from build123d import *

# Parameters (mm, degrees)
SKETCH1_R            = 21
BOSS_EXTRUDE1_DEPTH  = 3.5
SKETCH5_R            = 2.5
BOSS_EXTRUDE2_DEPTH  = 5
SKETCH6_R            = 5
SKETCH6_R_2          = 2.5
BOSS_EXTRUDE3_DEPTH  = 2.5
SKETCH7_R            = 17.5
BOSS_EXTRUDE4_DEPTH  = 0.75
SKETCH8_R            = 5
BOSS_EXTRUDE5_DEPTH  = 2.5
SKETCH10_R           = 1.125
SKETCH10_R_2         = 0.625
BOSS_EXTRUDE12_DEPTH = 0.5
CIRPATTERN1_COUNT    = 30


with BuildPart() as part:
    # Sketch1 → Boss-Extrude1 (new body)
    with BuildSketch(Plane(origin=(0, 0, 0), x_dir=(1, 0, 0), z_dir=(0, 1, 0))):
        with Locations(Location((0, 0, 0), (0, 0, 270))):
            Circle(SKETCH1_R)
    extrude(amount=BOSS_EXTRUDE1_DEPTH)

    # Sketch2 → Revolve3 (revolve)
    with BuildSketch(Plane.XY, mode=Mode.PRIVATE) as revolve3_sk:
        with BuildLine():
            Line((0, 3.5), (-20.5, 3.5))
            ThreePointArc((-20.5, 3.5), (-21.360863499, 9), (-20.5, 14.5))
            Line((-20.5, 14.5), (0, 14.5))
            Line((0, 14.5), (0, 3.5))
        make_face()
    revolve(revolve3_sk.sketch.rotate(Axis((0, 3.5, 0), (0, 1, 0)), 180), axis=Axis((0, 3.5, 0), (0, 1, 0)))

    # Sketch4 → Revolve4 (revolve)
    with BuildSketch(Plane.XY):
        with BuildLine():
            Line((0, 14.5), (21, 14.5))
            ThreePointArc((21, 14.5), (19.802282406, 20.151141203), (16, 24.5))
            Line((16, 24.5), (0, 24.5))
            Line((0, 24.5), (0, 14.5))
        make_face()
    revolve(axis=Axis((0, 14.5, 0), (0, 1, 0)))

    # Sketch5 → Boss-Extrude2 (add, symmetric)
    with BuildSketch(Plane.XY):
        with BuildLine():
            Line((0, 24.5), (10, 24.5))
            Line((10, 24.5), (10, 45.5))
            ThreePointArc((10, 45.5), (0, 55.5), (-10, 45.5))
            Line((-10, 45.5), (-10, 24.5))
            Line((-10, 24.5), (0, 24.5))
        make_face()
        with Locations((0, 45.5)):
            Circle(SKETCH5_R, mode=Mode.SUBTRACT)
    extrude(amount=BOSS_EXTRUDE2_DEPTH, both=True)

    # Sketch6 → Boss-Extrude3 (add, symmetric)
    with BuildSketch(Plane(origin=(0, 0, -5), x_dir=(-1, 0, 0), z_dir=(0, 0, -1))):
        with Locations(Location((0, 45.5, 0), (0, 0, 180))):
            Circle(SKETCH6_R)
        with Locations((0, 45.5)):
            Circle(SKETCH6_R_2, mode=Mode.SUBTRACT)
    extrude(amount=BOSS_EXTRUDE3_DEPTH, both=True)

    # Sketch7 → Boss-Extrude4 (add, symmetric)
    with BuildSketch(Plane.XZ):
        with Locations(Location((0, 0, 0), (0, 0, 90))):
            Circle(SKETCH7_R)
    extrude(amount=BOSS_EXTRUDE4_DEPTH, both=True)

    # Sketch8 → Boss-Extrude5 (add, symmetric)
    with BuildSketch(Plane(origin=(0, -0.75, 0), x_dir=(-1, 0, 0), z_dir=(0, -1, 0))):
        with Locations(Location((0, 0, 0), (0, 0, 90))):
            Circle(SKETCH8_R)
    extrude(amount=BOSS_EXTRUDE5_DEPTH, both=True)

    # Sketch10 → Boss-Extrude12 (add)
    with BuildSketch(Plane.XZ):
        with Locations(Location((19.148756021, 0, 0), (0, 0, 90))):
            Circle(SKETCH10_R)
        with Locations(Location((19.148756021, 0, 0), (0, 0, 270))):
            Circle(SKETCH10_R_2, mode=Mode.SUBTRACT)
    boss_extrude12 = extrude(amount=BOSS_EXTRUDE12_DEPTH)

    # CirPattern1: Boss-Extrude12 ×30 about axis
    cirpattern1_axis = Axis((0, 0, 0), (0, 1, 0))
    for i in range(1, CIRPATTERN1_COUNT):
        add(boss_extrude12.rotate(cirpattern1_axis, i * 360 / CIRPATTERN1_COUNT))


solid = part.part
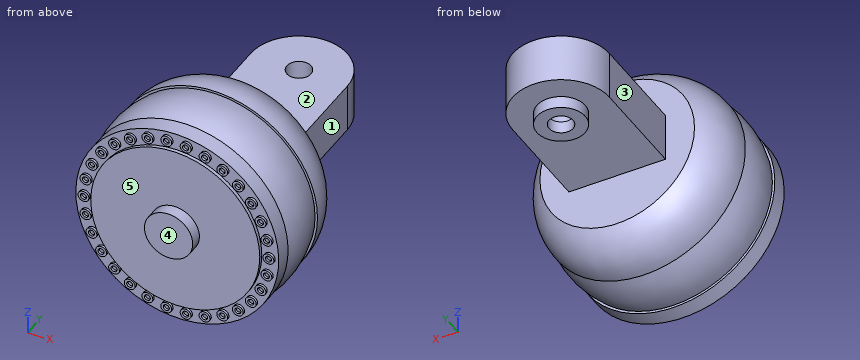
Model file for the job. Use its own axes, mm. Face numbers are marked on the shaded views. A direction names the side the tool comes from. Coordinates: 2 decimals unless noted, no trailing zeros. Write each loop counter-clockwise with the first axis right and the second up, starting at its lowest first coordinate (ties: lowest second). Pieces come first, ordered by that corner, then holes. Notation, with made-up numbers: (74, -6.5) - (112, -6.5) arc R23 cw to (112, 15.5) - close; hole circle Ø3 at (-18.5, 25.5). An arc over 180 degrees is marked (long way). Write each question's results on one line, items separated by ' | '. Start each with the question number.
1) 3-axis set-ups, long thin cutter, end or side, ignore diameter. For the marked faces 1, 2, 3, 4 and 5: which of +Z, -Z, +X, -X, +Y, -Y reach the whole face in a straight line?
2) Cut at A-A (y = 47). Write the cut outline in (x, z).
3) Flat gauge pins, fed straight in: P1, Ø1.6, axis at x = 17.49, z = 7.79, coming from the +Y side; P2, Ø1.4, axis at x = 19.15, z = 0, coming from the +Y side; P3, Ø4, axis at y = 30, z = 4.5, coming from the +X side. Where does each tip first touch, or does it go through?
4) Probe line 1 along X through (y, z) = (-0.1, 0); line 2 along X through (y, z) = (45.5, -1); line 3 along Y through (x, z) = (3.5, 15). List the from-to ranges inside material, lowest first. Write a range as from..to.
5) Cut at B-B (y = 33.5). Write the cut outline in (x, z).
Returned:
1) face 1: +Z, -Z, +X, +Y | face 2: +Z, +X, -X, +Y | face 3: +Z, -Z, -X, +Y | face 4: +Z, -Z, +X, -X, -Y | face 5: -Y
2) outline: (-9.89, -5) - (-4.77, -5) - (-4.77, -7.5) - (-2, -7.5) - (-2, 5) - (-9.89, 5) - close; (2, -7.5) - (4.77, -7.5) - (4.77, -5) - (9.89, -5) - (9.89, 5) - (2, 5) - close
3) P1: y = 22.37 | P2: y = 22.25 | P3: x = 10
4) line 1: -20.27..-19.77, -18.52..-18.02, -17.5..17.5, 18.02..18.52, 19.77..20.27 | line 2: -10..-2.5, 2.5..10 | line 3: -0.75..24.5
5) outline: (-10, -5) - (10, -5) - (10, 5) - (-10, 5) - close
